Work out the finished part from the listing and answer in its coordinate system (mm). Round coordinates to 2 decimals unless told otherwise and drop trailing zeros. Write each loop counter-clockwise with the first axis right and the second up, starting at its lowest first coordinate (ties: lowest second). Pieces come first, ordered by that corner, then holes. Notation, with made-up numbers: M 77.5,37 L 135.5,37 A9 cw 135.5,48 Z; hole C -24,40.5 d4. An arc over 180 degrees is marked long. Answer in a Markdown table with one row per item.
```python
from build123d import *

# Parameters (mm, degrees)
F1_DEPTH  = 3
F3_D      = 3.3
F5_D      = 5.5
F6_DEPTH  = 3.001
F7_R      = 0.6
F8_R      = 0.5
F10_D     = 3.3
F11_DEPTH = 3.001
F12_W     = 10.8
F12_H     = 28
F13_DEPTH = 3.001
F14_R     = 0.5


# Not quite as in the source:
# - a feature names something its author has since deleted; it is built from what else it names


with BuildPart() as f1:
    # F0 (on Top) → F1 (new body)
    with BuildSketch(Plane.XY):
        with BuildLine():
            Line((60, 55), (-60, 55))
            Line((-60, 55), (-60, -55))
            Line((-60, -55), (32, -55))
            Line((32, -55), (32, -45))
            ThreePointArc((32, -45), (40, -37), (48, -45))
            Line((48, -45), (48, -55))
            Line((48, -55), (60, -55))
            Line((60, -55), (60, 55))
        make_face()
    extrude(amount=F1_DEPTH)

    # F3 (through all)
    with Locations(Plane.XY.offset(3)):
        with Locations((-53, 27.5), (0, 48), (53, 27.5), (0, -48)):
            Hole(F3_D / 2)

    # F5 (through all)
    with Locations(Plane.XY.offset(3)):
        with Locations((-42.7202362838, 38.5875506155), (-42.7202362838, -32.9124493845), (28.7797637162, -32.9124493845), (28.7797637162, 38.5875506155)):
            Hole(F5_D / 2)

    # F4 (on face) → F6 (cut, through all)
    with BuildSketch(Plane.XY.offset(3)):
        with BuildLine():
            ThreePointArc((31.5297637162, 11.3375506155), (22.7429671518, 32.5507540511), (1.5297637162, 41.3375506155))
            Line((1.5297637162, 41.3375506155), (-15.4702362838, 41.3375506155))
            ThreePointArc((-15.4702362838, 41.3375506155), (-36.6834397194, 32.5507540511), (-45.4702362838, 11.3375506155))
            Line((-45.4702362838, 11.3375506155), (-45.4702362838, -5.6624493845))
            ThreePointArc((-45.4702362838, -5.6624493845), (-36.6834397194, -26.8756528201), (-15.4702362838, -35.6624493845))
            Line((-15.4702362838, -35.6624493845), (1.5297637162, -35.6624493845))
            ThreePointArc((1.5297637162, -35.6624493845), (22.7429671518, -26.8756528201), (31.5297637162, -5.6624493845))
            Line((31.5297637162, -5.6624493845), (31.5297637162, 11.3375506155))
        make_face()
    extrude(amount=-F6_DEPTH, mode=Mode.SUBTRACT)

    # F7
    f7_edges = [f1.edges().sort_by_distance(p)[0] for p in [
        (-60, 55, 1.5),
        (60, 55, 1.5),
        (60, -55, 1.5),
        (-60, -55, 1.5),
    ]]
    fillet(f7_edges, radius=F7_R)

    # F8
    f8_edges = [f1.edges().sort_by_distance(p)[0] for p in [
        (40, -37, 3),
        (-13.7, -55, 3),
    ]]
    fillet(f8_edges, radius=F8_R)

    # F10 (through all)
    with Locations(Plane.XY.offset(3)):
        with Locations((45.5, 10), (45.5, -30)):
            Hole(F10_D / 2)

    # F9 (on face) → F11 (cut, through all)
    with BuildSketch(Plane.XY.offset(3)):
        with BuildLine():
            Line((52.3, 3.75), (38.5, 3.75))
            ThreePointArc((38.5, 3.75), (36.3786796564, 2.8713203436), (35.5, 0.75))
            Line((35.5, 0.75), (35.5, -20.55))
            ThreePointArc((35.5, -20.55), (36.3786796564, -22.6713203436), (38.5, -23.55))
            Line((38.5, -23.55), (52.3, -23.55))
            ThreePointArc((52.3, -23.55), (54.4213203436, -22.6713203436), (55.3, -20.55))
            Line((55.3, -20.55), (55.3, 0.75))
            ThreePointArc((55.3, 0.75), (54.4213203436, 2.8713203436), (52.3, 3.75))
        make_face()
    extrude(amount=-F11_DEPTH, mode=Mode.SUBTRACT)

    # F12 (on face) → F13 (cut, through all)
    with BuildSketch(Plane.XY.offset(3)):
        with Locations((42.4, 36.5)):
            Rectangle(F12_W, F12_H)
    extrude(amount=-F13_DEPTH, mode=Mode.SUBTRACT)

    # F14
    f14_edges = [f1.edges().sort_by_distance(p)[0] for p in [
        (37, 22.5, 1.5),
        (37, 50.5, 1.5),
        (47.8, 50.5, 1.5),
        (47.8, 22.5, 1.5),
    ]]
    fillet(f14_edges, radius=F14_R)


solid = f1.part
```
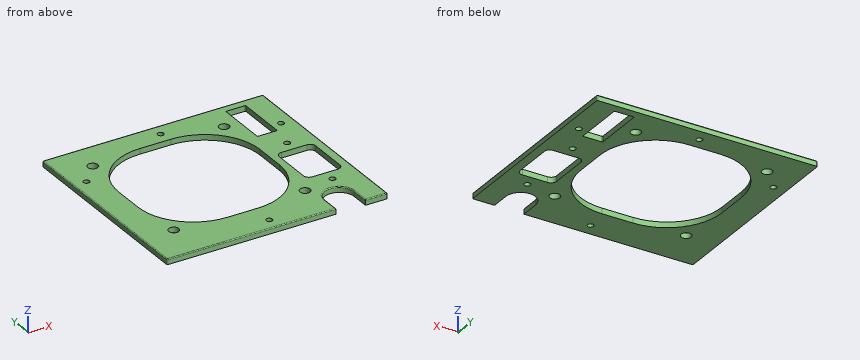
1. The part is cut by section B-B (x = -7). Determine the outline of the cut face in (y, z), plus the area to 3 significant figures.
Calculated:
| item | result |
|---|---|
| outline | M -55,0 L -35.66,0 L -35.66,3 L -54.5,3 A0.5 ccw -55,2.5 Z; M 41.34,0 L 55,0 L 55,2.5 A0.5 ccw 54.5,3 L 41.34,3 Z |
| area | 98.9 mm² |
2. The part is cut by section D-D (y = 10). Determine the outline of the cut face in (x, z), plus the area to 3 significant figures.
Calculated:
| item | result |
|---|---|
| outline | M -60,0 L -45.47,0 L -45.47,3 L -59.5,3 A0.5 ccw -60,2.5 Z; M 31.53,0 L 43.85,0 L 43.85,3 L 31.53,3 Z; M 47.15,0 L 60,0 L 60,2.5 A0.5 ccw 59.5,3 L 47.15,3 Z |
| area | 119 mm² |
3. The part is cut by section A-A (y = -48). Determine the outline of the cut face in (x, z), plus the area to 3 significant figures.
Calculated:
| item | result |
|---|---|
| outline | M -60,0 L -1.65,0 L -1.65,3 L -59.5,3 A0.5 ccw -60,2.5 Z; M 1.65,0 L 32,0 L 32,2.5 A0.5 ccw 31.5,3 L 1.65,3 Z; M 48,0 L 60,0 L 60,2.5 A0.5 ccw 59.5,3 L 48.5,3 A0.5 ccw 48,2.5 Z |
| area | 302 mm² |
4. The part is cut by section C-C (x = 40). Determine the outline of the cut face in (y, z).
Calculated:
| item | result |
|---|---|
| outline | M -37,0 L -23.55,0 L -23.55,3 L -36.5,3 A0.5 ccw -37,2.5 Z; M 3.75,0 L 22.5,0 L 22.5,3 L 3.75,3 Z; M 50.5,0 L 55,0 L 55,2.5 A0.5 ccw 54.5,3 L 50.5,3 Z |
5. Consider line 1 along Y through (x, z) = (-7.5, 0.6); line 2 along Y through (x, z) = (-53, 1.65); line 3 along X through (y, z) = (-21, 0.3). Determine where each line is inside the solid, lowest interval first. Write a range as from..to.
Calculated:
| item | result |
|---|---|
| line 1 | y = -55..-35.66, 41.34..55 |
| line 2 | y = -55..25.85, 29.15..55 |
| line 3 | x = -60..-41.25, 27.31..35.53, 55.27..60 |
6. Given pin 1 (1.5 mm diameter, centred on x = 44.5, z = 1, fed in from -Y), flat-ended and moving along its own axis, determine where the tip first touches the part or whether it passes through.
Calculated:
| item | result |
|---|---|
| pin 1 | stops at y = -38.96 |
